Geometry check sheet. Reference: drawing and pictorial views, mm from the part's lowest x, y, z. Coordinates: 2 decimals unless noted, no trailing zeros. Write each loop counter-clockwise with the first axis right and the second up, starting at its lowest first coordinate (ties: lowest second). Pieces come first, ordered by that corner, then holes.
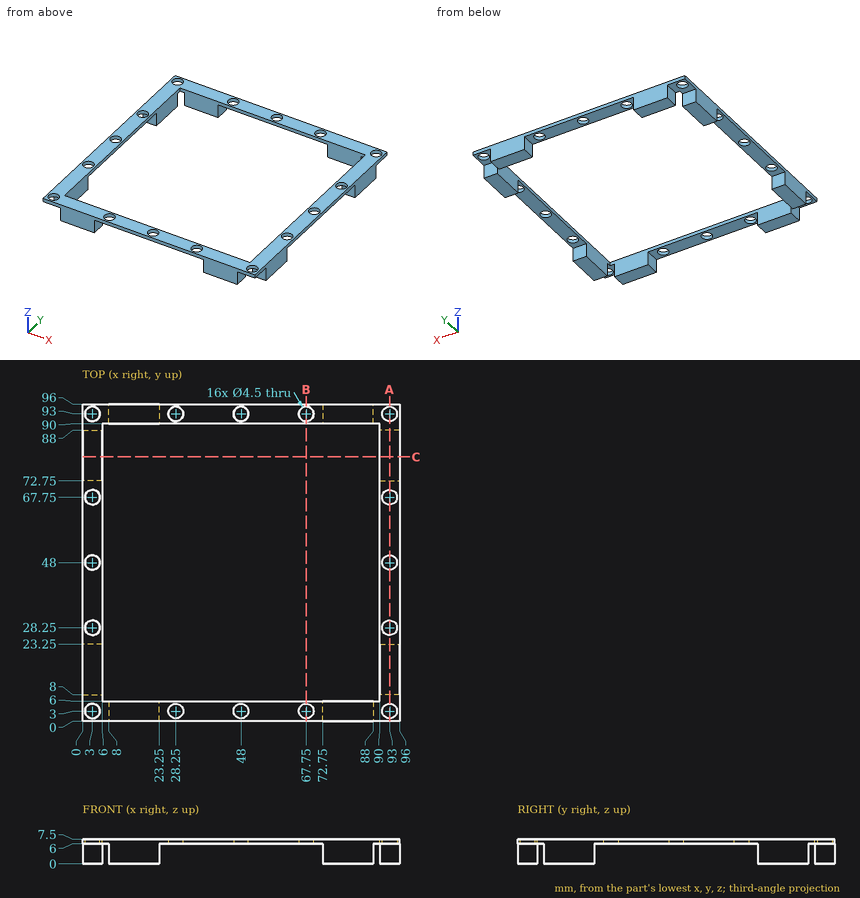
1. Material ranges on L1, parallel to Y at x = 67.75, z = 6.6; L2, parallel to Y at x = 93, z = 6.95; L3, parallel to X at y = 19, z = 0.5, recorded low to high.
2. Sectioned sample at B-B, the plane x = 67.75. Record the boundary of the cut face in (y, z).
3. Sectioned sample at C-C, the plane y = 80. Record the boundary of the cut face in (x, z), and give its area (3 significant figures).
4. Sectioned sample at A-A, the plane x = 93. Give the number of separate pieces and of enclosed holes in the cut face, and give its area (3 significant figures).
5. Gauge pin test, flat ends, axial feed: P1, Ø6, axis at x = 3, y = 67.75, coming from the -Z side; P2, Ø3, axis at x = 3, z = 2.5, coming from the +Y side; P3, Ø4, axis at x = 93, y = 67.75, coming from the -Z side; P4, Ø1.8, axis at x = 3, z = 2, coming from the -Y side. Record the tip position at first contact, or that the pin passes through.
Outcome:
1. L1: y = 0 to 0.75, 5.25 to 6, 90 to 90.75, 95.25 to 96
1. L2: y = 0 to 0.75, 5.25 to 26, 30.5 to 45.75, 50.25 to 65.5, 70 to 90.75, 95.25 to 96
1. L3: x = 0 to 6, 90 to 96
2. outline: (0, 6) - (0.75, 6) - (0.75, 7.5) - (0, 7.5) - close; (5.25, 6) - (6, 6) - (6, 7.5) - (5.25, 7.5) - close; (90, 6) - (90.75, 6) - (90.75, 7.5) - (90, 7.5) - close; (95.25, 6) - (96, 6) - (96, 7.5) - (95.25, 7.5) - close
3. outline: (0, 0) - (6, 0) - (6, 7.5) - (0, 7.5) - close; (90, 0) - (96, 0) - (96, 7.5) - (90, 7.5) - close
3. area: 90.0 mm2
4. separate pieces: 6
4. enclosed holes: 0
4. area: 293 mm2
5. P1: stops at z = 6
5. P2: stops at y = 88
5. P3: passes through
5. P4: stops at y = 8
